Autodesk Inventor part; units mm, degrees
ref_plane "YZ Plane" through (0, 0, 0) normal (1, 0, 0) x (0, 1, 0)
ref_plane "XZ Plane" through (0, 0, 0) normal (0, 1, 0) x (-1, 0, 0)
ref_plane "XY Plane" through (0, 0, 0) normal (0, 0, 1) x (1, 0, 0)
sketch "Sketch1" plane through (0, 0, 0) normal (0, 1, 0) x (-1, 0, 0)
  line L0 (9.8, 0) -> (-9.8, 0)
  line L1 (0, -5.6) -> (0, 5.6)
  line L2 (-7, 4) -> (7, 4)
  line L3 (7, 4) -> (7, -4)
  line L4 (7, -4) -> (-7, -4)
  line L5 (-7, -4) -> (-7, 4)
  line L6 (-7, 4) -> (7, -4) construction
  line L7 (7, 4) -> (-7, -4) construction
  point P0 (0, 0)
  dimension "d0" = 14
  dimension "d1" = 8
extrude "Extrusion1" add sketch "Sketch1" along normal blind 3
sketch "Sketch2" plane through (0, 3, 0) normal (0, 1, 0) x (1, 0, 0)
  line L0 (-7, 4) -> (-7, -4)
  line L1 (7, -4) -> (7, 4)
  line L2 (-7, -4) -> (7, -4)
  line L3 (7, -4) -> (7, -2)
  line L4 (7, -2) -> (-7, -2)
  line L5 (-7, -2) -> (-7, -4)
  point P0 (0, 0)
  point P1 (-7, -2)
  dimension "d4" = 2
extrude "Extrusion2" add sketch "Sketch2" along normal blind 21
sketch "Sketch3" plane through (7, 3, 2) normal (0, 0, -1) x (-1, 0, 0)
  line L0 (0, -3) -> (0, 21)
  line L1 (14, -3) -> (14, 21)
  line L2 (0, 21) -> (14, 21)
  line L3 (14, 21) -> (14, 18)
  line L4 (14, 18) -> (0, 18)
  line L5 (0, 18) -> (0, 21)
  point P0 (7, -3)
  point P1 (0, 18)
  dimension "d7" = 3
extrude "Extrusion3" add sketch "Sketch3" along normal up to surface (6 mm away)
properties part number "uchwyt_krancowka_alternatywa_2"
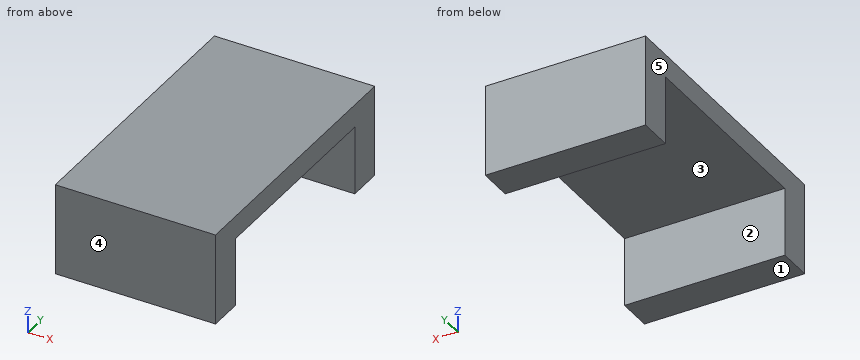
The listing builds one solid part. Answer for the finished solid, in the listing's coordinates (mm). Face numbers are marked on the shaded views. A direction names the side the tool comes from. Give positions to 0.01 mm unless a question says otherwise; leave off trailing zeros. Write each loop counter-clockwise with the first axis right and the second up, starting at its lowest first coordinate (ties: lowest second). Pieces come first, ordered by that corner, then holes. Notation, with made-up numbers: (-7.5, -4) -> (44.5, -4) arc R11 ccw to (44.5, 11) -> close; hole circle Ø4 at (2.5, -16.75). An arc over 180 degrees is marked (long way). One line per question, with ' | ' between items. Start each with the question number.
1. For a pull along Y with two mould halves and no side action, classify the marked faces 3, 4 and 5 as pulls with the +Y half, pulls with the -Y half, needs draft (parallel to the pull), parting line crosses it, or undercut.
2. Given pin 1 Ø5 at (x, y) = (1, 10.5) entering from -Z, flat-ended and moving along its own axis, determine where the tip first touches the part or whether it passes through.
3. Section C-C (y = 16.75) is taken. Determine the outline of the cut face in (x, z).
4. Section B-B (x = 1.75) is taken. Determine the outline of the cut face in (y, z), plus the area to 3 significant figures.
5. Find the intervals of material crossed by probe 1 along Y at (x, z) = (6.75, 0.25); probe 2 along Z at (x, y) = (-0.25, 15.75), in increasing order.
6. For the marked faces 1 and 2, determine the directions among +Z, -Z, +X, -X, +Y, -Y from which every point of the face is accessible in a straight line to the end or side of a thin tool.
7. Section A-A (z = -2.75) is taken. Determine the outline of the cut face in (x, y), plus the area to 3 significant figures.
Response values:
1) face 3: undercut | face 4: pulls with the -Y half | face 5: needs draft
2) pin 1: z = 2
3) outline: (-7, 2) -> (7, 2) -> (7, 4) -> (-7, 4) -> close
4) outline: (0, -4) -> (3, -4) -> (3, 2) -> (21, 2) -> (21, -4) -> (24, -4) -> (24, 4) -> (0, 4) -> close | area: 84.0 mm2
5) probe 1: 0 to 3, 21 to 24 | probe 2: 2 to 4
6) face 1: -Z, +X, -X, +Y, -Y | face 2: -Z, +X, -X
7) outline: (-7, 0) -> (7, 0) -> (7, 3) -> (-7, 3) -> close; (-7, 21) -> (7, 21) -> (7, 24) -> (-7, 24) -> close | area: 84.0 mm2
